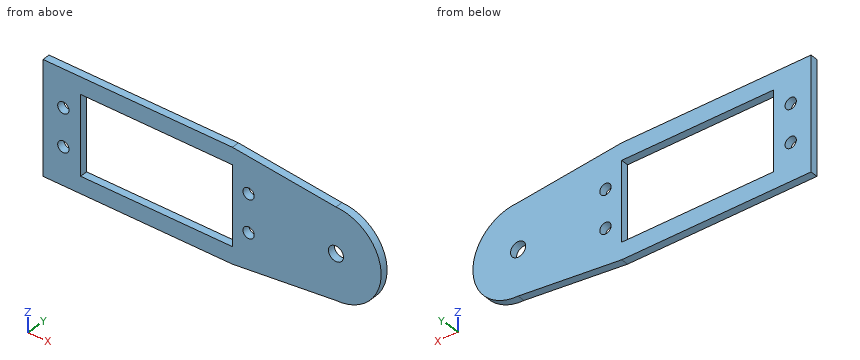
from build123d import *

# Parameters (mm, degrees)
SKETCH_1_R         = 1.5
SKETCH_1_R_2       = 2
SKETCH_1_W         = 40.3
SKETCH_1_H         = 21
EXTRUDE_1090_DEPTH = 2


with BuildPart() as part:
    # Эскиз1 → Extrude 1090 (new body)
    with BuildSketch(Plane(origin=(0, 0, 0), x_dir=(1, 0, 0), z_dir=(0, 1, 0))):
        with BuildLine():
            Line((0, 15), (50.3, 15))
            Line((50.3, 15), (77.8, 12))
            ThreePointArc((77.8, 12), (89.8, 0), (77.8, -12))
            Line((77.8, -12), (50.3, -15))
            Line((50.3, -15), (0, -15))
            Line((0, -15), (0, 15))
        make_face()
        with Locations(Location((5.4, -5, 0), (0, 0, 270))):
            Circle(SKETCH_1_R, mode=Mode.SUBTRACT)
        with Locations(Location((5.4, 5, 0), (0, 0, 270))):
            Circle(SKETCH_1_R, mode=Mode.SUBTRACT)
        with Locations(Location((54.6, -5, 0), (0, 0, 270))):
            Circle(SKETCH_1_R, mode=Mode.SUBTRACT)
        with Locations(Location((54.6, 5, 0), (0, 0, 270))):
            Circle(SKETCH_1_R, mode=Mode.SUBTRACT)
        with Locations(Location((77.8, 0, 0), (0, 0, 270))):
            Circle(SKETCH_1_R_2, mode=Mode.SUBTRACT)
        with Locations((30.15, 0)):
            Rectangle(SKETCH_1_W, SKETCH_1_H, mode=Mode.SUBTRACT)
    extrude(amount=EXTRUDE_1090_DEPTH)


solid = part.part
Input: part model. Units: mm. Frame: model coordinates. Coordinates: 2 decimals unless noted, no trailing zeros. Loops run counter-clockwise (first coordinate to the right, second up) from the corner with the lowest first, then second, coordinate; pieces in that order, holes last. Notation, with made-up numbers: (18.5, 35) -> (60.5, 35) arc R33 cw to (60.5, 69) -> close; hole circle Ø2 at (81.5, 67.25). An arc over 180 degrees is marked (long way). Write each question's results on one line, items separated by ' | '. Start each with the question number.
Q1. Section B-B, the plane y = 0.5. Return the cut outline in (x, z).
Q2. Section D-D, the plane x = 5.4. Return the cut outline in (y, z), plus the area to 3 significant figures.
Q3. Pin query (flat end, axial travel): pin 1 (2.5 mm diameter, centred on x = 5.4, z = -5, fed in from +Y). Return the tip coordinate at first contact, or that it passes through.
Q4. Section A-A, the plane x = 18.5. Return the cut outline in (y, z).
Q5. Section C-C, the plane z = 0. Return the cut outline in (x, y).
Q6. Ray query, line 1 (X direction, y = 0.7, z = 0); line 2 (X direction, y = 1.45, z = -5); line 3 (Z direction, x = 37, y = 1.6). Return the intervals inside material, ascending. Write a range as from..to.
Found:
1) outline: (0, -15) -> (50.3, -15) -> (77.8, -12) arc R12 ccw to (77.8, 12) -> (50.3, 15) -> (0, 15) -> close; hole circle Ø3 at (5.4, -5); hole circle Ø3 at (5.4, 5); hole (10, -10.5) -> (50.3, -10.5) -> (50.3, 10.5) -> (10, 10.5) -> close; hole circle Ø3 at (54.6, -5); hole circle Ø3 at (54.6, 5); hole circle Ø4 at (77.8, 0)
2) outline: (0, -15) -> (2, -15) -> (2, -6.5) -> (0, -6.5) -> close; (0, -3.5) -> (2, -3.5) -> (2, 3.5) -> (0, 3.5) -> close; (0, 6.5) -> (2, 6.5) -> (2, 15) -> (0, 15) -> close | area: 48.0 mm2
3) pin 1: through
4) outline: (0, -15) -> (2, -15) -> (2, -10.5) -> (0, -10.5) -> close; (0, 10.5) -> (2, 10.5) -> (2, 15) -> (0, 15) -> close
5) outline: (0, 0) -> (10, 0) -> (10, 2) -> (0, 2) -> close; (50.3, 0) -> (75.8, 0) -> (75.8, 2) -> (50.3, 2) -> close; (79.8, 0) -> (89.8, 0) -> (89.8, 2) -> (79.8, 2) -> close
6) line 1: 0..10, 50.3..75.8, 79.8..89.8 | line 2: 0..3.9, 6.9..10, 50.3..53.1, 56.1..88.71 | line 3: -15..-10.5, 10.5..15
